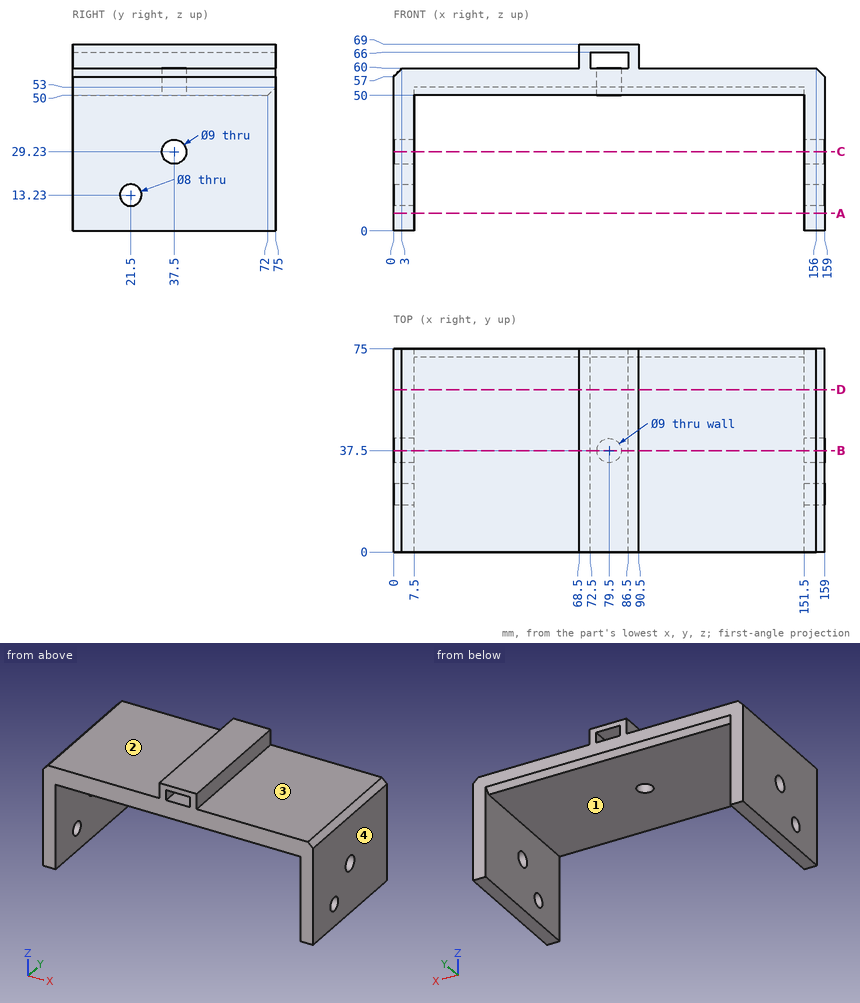
Geometry check sheet. Reference: drawing and pictorial views, mm from the part's lowest x, y, z. A direction names the side the tool comes from. Coordinates: 2 decimals unless noted, no trailing zeros. Order: outer loops, then holes, each group sorted by start corner. A loop starts at its lowest first (then second) coordinate and runs counter-clockwise, first axis right, second up. Notation, with made-up numbers: M -23.75,48 L -3.75,48 A25 cw -3.75,71 Z; hole C -29,34.5 d7. An arc over 180 degrees is marked long. Return JSON: item names as keys, results as strings.
1) Access from +Z, -Z, +X, -X, +Y, -Y to the whole of each face (thin tool, end or side, straight path). Record for the marked faces 1, 2, 3 and 4.
Answer list:
{"face 1": "-Z, +Y, -Y", "face 2": "+Z, -X, +Y, -Y", "face 3": "+Z, +X, +Y, -Y", "face 4": "+Z, -Z, +X, +Y, -Y"}
2) Cross-section at D-D, the plane y = 60. Record the boundary of the cut face in (x, z).
Answer list:
{"outline": "M 0,0 L 7.5,0 L 7.5,50 L 151.5,50 L 151.5,0 L 159,0 L 159,57 L 156,60 L 90.5,60 L 90.5,69 L 68.5,69 L 68.5,60 L 3,60 L 0,57 Z; hole M 72.5,60 L 86.5,60 L 86.5,66 L 72.5,66 Z"}
3) Cross-section at C-C, the plane z = 29.23. Record the boundary of the cut face in (x, y), and give its area (3 significant figures).
Answer list:
{"outline": "M 0,0 L 7.5,0 L 7.5,33 L 0,33 Z; M 0,42 L 7.5,42 L 7.5,75 L 0,75 Z; M 151.5,0 L 159,0 L 159,33 L 151.5,33 Z; M 151.5,42 L 159,42 L 159,75 L 151.5,75 Z", "area": "990 mm2"}
4) Cross-section at B-B, the plane y = 37.5. Count the separate pieces of the cut face and the enclosed holes in it, and give its area (3 significant figures).
Answer list:
{"separate pieces": "3", "enclosed holes": "0", "area": "2,220 mm2"}
5) Cross-section at A-A, the plane z = 6.5. Record the boundary of the cut face in (x, y).
Answer list:
{"outline": "M 0,0 L 7.5,0 L 7.5,75 L 0,75 Z; M 151.5,0 L 159,0 L 159,75 L 151.5,75 Z"}
6) Thickness scan on L1, parallel to X at y = 66, z = 65; L2, parallel to X at y = 64.5, z = 8; L3, parallel to Z at x = 84, y = 33.5. Record the ranges inside material, lowest first. Write a range as [from, to].
Answer list:
{"L1": "[68.5, 72.5], [86.5, 90.5]", "L2": "[0, 7.5], [151.5, 159]", "L3": "[50, 60], [66, 69]"}
7) Gauge pin test, flat ends, axial feed: pin 1 (4 mm diameter, centred on x = 84.5, y = 36.5, fed in from -Z); pin 2 (10.5 mm diameter, centred on y = 37.5, z = 29.23, fed in from +X); pin 3 (2.5 mm diameter, centred on y = 43.5, z = 63.5, fed in from +X); pin 4 (1.8 mm diameter, centred on y = 24.5, z = 62.5, fed in from -X). Record the tip position at first contact, or that the pin passes through.
Answer list:
{"pin 1": "z = 50", "pin 2": "x = 159", "pin 3": "x = 90.5", "pin 4": "x = 68.5"}
